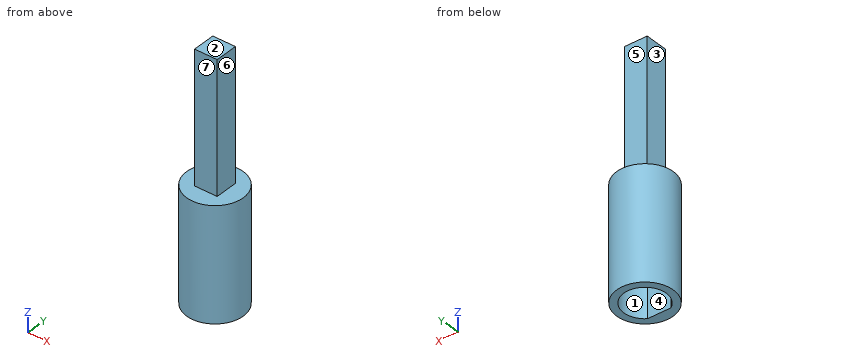
from build123d import *

# Parameters (mm, degrees)
SKETCH1_R           = 4
BOSS_EXTRUDE1_DEPTH = 16
CUT_EXTRUDE3_DEPTH  = 14
SKETCH6_W           = 3.2
SKETCH6_H           = 3.2
BOSS_EXTRUDE2_DEPTH = 18.5


with BuildPart() as part:
    # Sketch1 → Boss-Extrude1 (new body)
    with BuildSketch(Plane.XY):
        Circle(SKETCH1_R)
    extrude(amount=BOSS_EXTRUDE1_DEPTH)

    # Sketch3 → Cut-Extrude3 (cut)
    with BuildSketch(Plane(origin=(0, 0, 0), x_dir=(-1, 0, 0), z_dir=(0, 0, -1))):
        with BuildLine():
            Line((-1.658312395, -2.5), (1.658312395, -2.5))
            ThreePointArc((1.658312395, -2.5), (0, 3), (-1.658312395, -2.5))
        make_face()
    extrude(amount=-CUT_EXTRUDE3_DEPTH, mode=Mode.SUBTRACT)

    # Sketch6 → Boss-Extrude2 (add)
    with BuildSketch(Plane.XY.offset(16)):
        Rectangle(SKETCH6_W, SKETCH6_H)
    extrude(amount=BOSS_EXTRUDE2_DEPTH)


solid = part.part
Check sheet for the modelled part. Datum: model origin and axes. Units: mm. Face numbers are marked on the shaded views. A direction names the side the tool comes from. Round coordinates to 2 decimals unless told otherwise and drop trailing zeros. Order: outer loops, then holes, each group sorted by start corner. A loop starts at its lowest first (then second) coordinate and runs counter-clockwise, first axis right, second up. Notation, with made-up numbers: M 4.25,55 L 43.25,55 A13 ccw 43.25,69 Z; hole C -19,9 d1. An arc over 180 degrees is marked long. One line per item, written item: value. Start each with the question number.
1. Section check D-D on y = 2. Enter the section's corners in (x, z), and give its area (3 significant figures).
2. Section check C-C on z = 4. Enter the section's corners in (x, y).
3. Release check for a two-part mould opening along X. For the marked faces 1, 2, 3 and 4 record: released by +X, released by -X, zero draft, split by the parting line, or undercut.
4. Section check A-A on y = 0. Enter the section's corners in (x, z).
5. Scan lines: line 1 along Y through (x, z) = (0, 6.75); line 2 along X through (y, z) = (-1, 23); line 3 along Z through (x, y) = (2, -1). Record each from-to range of solid material in increasing order.
6. Access from +Z, -Z, +X, -X, +Y, -Y to the whole of each face (thin tool, end or side, straight path). Record for the marked faces 5, 6 and 7.
7. Gauge pin test, flat ends, axial feed: P1, Ø4, axis at y = -2.5, z = 14.5, coming from the -X side; P2, Ø1.6, axis at y = -0.5, z = 23, coming from the -X side; P3, Ø2, axis at y = 0.5, z = 10.5, coming from the +X side; P4, Ø1.5, axis at x = -0.5, y = -3, coming from the +Z side. Record the tip position at first contact, or that the pin passes through.
8. Section check B-B on x = 0. Enter the section's corners in (y, z).
Results found:
1. outline: M -3.46,0 L -2.24,0 L -2.24,14 L 2.24,14 L 2.24,0 L 3.46,0 L 3.46,16 L -3.46,16 Z
1. area: 48.2 mm^2
2. outline: C 0,0 d8; hole M -1.66,-2.5 L 1.66,-2.5 A3 ccw long Z
3. face 1: undercut
3. face 2: zero draft
3. face 3: released by -X
3. face 4: undercut
4. outline: M -4,0 L -3,0 L -3,14 L 3,14 L 3,0 L 4,0 L 4,16 L 1.6,16 L 1.6,34.5 L -1.6,34.5 L -1.6,16 L -4,16 Z
5. line 1: -4 to -2.5, 3 to 4
5. line 2: -1.6 to 1.6
5. line 3: 14 to 16
6. face 5: +Z, +X, -X, +Y
6. face 6: +Z, +X, +Y, -Y
6. face 7: +Z, +X, -X, -Y
7. P1: x = -3.97
7. P2: x = -1.6
7. P3: x = 4
7. P4: z = 16
8. outline: M -4,0 L -2.5,0 L -2.5,14 L 3,14 L 3,0 L 4,0 L 4,16 L 1.6,16 L 1.6,34.5 L -1.6,34.5 L -1.6,16 L -4,16 Z
